Could you check a few things on this model? Use its own coordinates, in mm. Round coordinates to 2 decimals unless told otherwise and drop trailing zeros. Loops run counter-clockwise (first coordinate to the right, second up) from the corner with the lowest first, then second, coordinate; pieces in that order, holes last. Notation, with made-up numbers: (-27, 46.5) -> (20, 46.5) arc R11 ccw to (20, 54.5) -> close; hole circle Ø5 at (28, 18). An arc over 180 degrees is marked (long way). One line per item, written item: value.
Autodesk Inventor part; units mm, degrees
ref_plane "YZ Plane" through (0, 0, 0) normal (1, 0, 0) x (0, 1, 0)
ref_plane "XZ Plane" through (0, 0, 0) normal (0, 1, 0) x (-1, 0, 0)
ref_plane "XY Plane" through (0, 0, 0) normal (0, 0, 1) x (1, 0, 0)
sketch "Sketch1" plane through (0, 0, 0) normal (1, 0, 0) x (0, 1, 0)
  circle A0 centre (0, 0) radius 6.35
  circle A1 centre (-44.45, 44.45) radius 1.905
  arc A2 (-40.1924, 49.1612) -> (-49.1612, 40.1924) centre (-44.45, 44.45) ccw
  arc A3 (-7.0668, -6.3864) -> (6.3864, 7.0668) centre (0, 0) ccw
  line L0 (0, 0) -> (0, -9.525) construction
  line L1 (0, 0) -> (-44.45, 44.45) construction
  line L2 (0, 0) -> (-44.45, -44.45) construction
  line L3 (0, 0) -> (-64.9365, 0) construction
  line L4 (-44.45, 44.45) -> (-48.9401, 48.9401) construction
  circle A4 centre (-8.9803, 8.9803) radius 1.5875
  line L5 (-49.1612, 40.1924) -> (-7.0668, -6.3864)
  line L6 (6.3864, 7.0668) -> (-40.1924, 49.1612)
  dimension "d0" = 12.7
  dimension "d1" = 3.81
  dimension "d10" = 12.7
  dimension "d15" = 88.9
  dimension "d16" = 3.175
  dimension "d17" = 12.7
  dimension "d18" = 9.525
extrude "Extrusion1" add sketch "Sketch1" along normal blind 4.7625
properties part number "torque arm"
(1) If we section it at C-C, the plane x = 3.65: Give the number of separate pieces and of enclosed holes in the cut face, then the cut area to 3 significant figures.
Recorded:
separate pieces: 1
enclosed holes: 3
area: 1,060 mm²
(2) Thinking about a two-plate mould opening in Z: for faces 1 (the face through (2.348, 6.886, -6.581)), 2 (the face through (2.348, -9.187, 7.406)), 3 (the face through (2.35, -16.58, 27.82)), which applies, released by +Z, released by -Z, zero draft, split by the parting line, or undercut?
Recorded:
face 1: split by the parting line
face 2: undercut
face 3: released by +Z
(3) If we section it at B-B, the plane z = -3.5: Please give me the cut outline in (x, y), then the cut area to 3 significant figures.
Recorded:
outline: (0, -9.68) -> (4.76, -9.68) -> (4.76, -5.3) -> (0, -5.3) -> close; (0, 5.3) -> (4.76, 5.3) -> (4.76, 8.86) -> (0, 8.86) -> close
area: 37.8 mm²
(4) If we section it at D-D, the plane y = -30: Please give me the cut outline in (x, z).
Recorded:
outline: (0, 18.99) -> (4.76, 18.99) -> (4.76, 39.95) -> (0, 39.95) -> close
(5) I'm going to push flat-ended pins straight in: pin 1 Ø1 at (x, z) = (4, 11) entering from -Y; pin 2 Ø2.5 at (y, z) = (-44.45, 44.45) entering from +X; pin 3 Ø1.5 at (x, z) = (2.5, 29) entering from +Y; pin 4 Ø1 at (x, y) = (2.5, -5) entering from -Z (3 decimals). Where does each tip first touch, or does it pass through?
Recorded:
pin 1: y = -23.23
pin 2: through
pin 3: y = -17.05
pin 4: z = -8.395
(6) If I drill on L1, parallel to Y at x = 1.8, z = 45; L2, parallel to Z at x = 2.95, y = 0 (3 decimals); L3, parallel to Z at x = 3.5, y = -44.45 (3 decimals), over which ranges is the centre line in solid material (lowest first)?
Recorded:
L1: -50.78 to -46.27, -42.63 to -35.59
L2: -9.525 to -6.35, 6.35 to 12.838
L3: 34.979 to 42.545, 46.355 to 50.8
